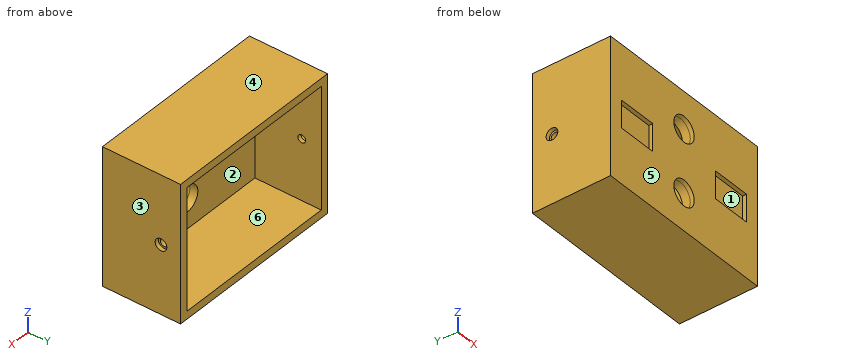
```python
from build123d import *

# Parameters (mm, degrees)
F0_W      = 47
F0_H      = 35
F1_DEPTH  = 19
F2_T      = -2
F3_R      = 3.25
F4_DEPTH  = 19.001
F1_FACE_W = 47
F1_FACE_H = 35
F1_FACE_R = 3.25
F5_DEPTH  = 1
F7_R      = 1
F8_DEPTH  = 47.001
F9_R      = 1.5
F10_DEPTH = 1
F11_R     = 1.5
F12_DEPTH = 1
F13_W     = 10
F13_H     = 7
F14_DEPTH = 1


with BuildPart() as f1:
    # F0 (on Front) → F1 (new body)
    with BuildSketch(Plane.XZ):
        Rectangle(F0_W, F0_H)
    extrude(amount=F1_DEPTH)

    # F2
    f2_openings = [f1.faces().sort_by_distance(p)[0] for p in [
        (0, 0, 0),
    ]]
    offset(amount=F2_T, openings=f2_openings)

    # F3 (on face) → F4 (cut, through all)
    with BuildSketch(Plane.XZ.offset(19)):
        with Locations((0, 8)):
            Circle(F3_R)
        with Locations((0, -8)):
            Circle(F3_R)
    extrude(amount=-F4_DEPTH, mode=Mode.SUBTRACT)

    # F1_face (on face) → F5 (join)
    with BuildSketch(Plane.XZ.offset(19)):
        Rectangle(F1_FACE_W, F1_FACE_H)
        with Locations((0, -8)):
            Circle(F1_FACE_R, mode=Mode.SUBTRACT)
        with Locations((0, 8)):
            Circle(F1_FACE_R, mode=Mode.SUBTRACT)
    extrude(amount=F5_DEPTH)

    # F7 (on face) → F8 (cut, through all)
    with BuildSketch(Plane(origin=(-23.5, 0, 0), x_dir=(0, -1, 0), z_dir=(-1, 0, 0))):
        with Locations((5, 0)):
            Circle(F7_R)
    extrude(amount=-F8_DEPTH, mode=Mode.SUBTRACT)

    # F9 (on face) → F10 (cut)
    with BuildSketch(Plane(origin=(-23.5, 0, 0), x_dir=(0, -1, 0), z_dir=(-1, 0, 0))):
        with Locations((5, 0)):
            Circle(F9_R)
    extrude(amount=-F10_DEPTH, mode=Mode.SUBTRACT)

    # F11 (on face) → F12 (cut)
    with BuildSketch(Plane.YZ.offset(23.5)):
        with Locations((-5, 0)):
            Circle(F11_R)
    extrude(amount=-F12_DEPTH, mode=Mode.SUBTRACT)

    # F13 (on face) → F14 (cut)
    with BuildSketch(Plane.XZ.offset(20)):
        with Locations((-15, 0)):
            Rectangle(F13_W, F13_H)
        with Locations((15, 0)):
            Rectangle(F13_W, F13_H)
    extrude(amount=-F14_DEPTH, mode=Mode.SUBTRACT)


solid = f1.part
```
Can you work these out from the model? Positions are in its coordinate system, mm. Face numbers are marked on the shaded views. A direction names the side the tool comes from. Coordinates: 2 decimals unless noted, no trailing zeros. Write each loop counter-clockwise with the first axis right and the second up, starting at its lowest first coordinate (ties: lowest second). Pieces come first, ordered by that corner, then holes. Notation, with made-up numbers: (72.25, -1.5) - (93.25, -1.5) arc R18 cw to (93.25, 2.5) - close; hole circle Ø3 at (-7.75, 39). An arc over 180 degrees is marked (long way). Return JSON: item names as keys, results as strings.
Q1. Please list where these lines run through material, in increasing order: L1, parallel to Z at x = -5.5, y = -2.25; L2, parallel to Z at x = 22.15, y = -5; L3, parallel to X at y = -12.75, z = -7. Write a range as from..to.
Computed values:
{"L1": "z = -17.5..-15.5, 15.5..17.5", "L2": "z = -17.5..-1, 1..17.5", "L3": "x = -23.5..-21.5, 21.5..23.5"}
Q2. If we section it at A-A (y = -5): Please give me the cut outline in (x, z), then the cut area to 3 significant figures.
Computed values:
{"outline": "(-23.5, -17.5) - (23.5, -17.5) - (23.5, -1.5) - (22.5, -1.5) - (22.5, -1) - (21.5, -1) - (21.5, -15.5) - (-21.5, -15.5) - (-21.5, -1) - (-22.5, -1) - (-22.5, -1.5) - (-23.5, -1.5) - close; (-23.5, 1.5) - (-22.5, 1.5) - (-22.5, 1) - (-21.5, 1) - (-21.5, 15.5) - (21.5, 15.5) - (21.5, 1) - (22.5, 1) - (22.5, 1.5) - (23.5, 1.5) - (23.5, 17.5) - (-23.5, 17.5) - close", "area": "302 mm2"}
Q3. I'm going to push flat-ended pins straight in: pin 1 Ø2.5 at (y, z) = (-5, 0) entering from -X; pin 2 Ø2.5 at (y, z) = (-5, 0) entering from +X; pin 3 Ø2 at (x, z) = (16.5, -1.5) entering from -Y; pin 4 Ø2 at (x, z) = (-1.5, 6.5) entering from -Y. Where does each tip first touch, or does it pass through?
Computed values:
{"pin 1": "stops at x = -22.5", "pin 2": "stops at x = 22.5", "pin 3": "stops at y = -19", "pin 4": "passes through"}
Q4. If we section it at D-D (z = 8): Please give me the cut outline in (x, y).
Computed values:
{"outline": "(-23.5, -20) - (-3.25, -20) - (-3.25, -17) - (-21.5, -17) - (-21.5, 0) - (-23.5, 0) - close; (3.25, -20) - (23.5, -20) - (23.5, 0) - (21.5, 0) - (21.5, -17) - (3.25, -17) - close"}
Q5. If we section it at C-C (z = 2.5): Please give me the cut outline in (x, y), then the cut area to 3 significant figures.
Computed values:
{"outline": "(-23.5, -20) - (-20, -20) - (-20, -19) - (-10, -19) - (-10, -20) - (10, -20) - (10, -19) - (20, -19) - (20, -20) - (23.5, -20) - (23.5, 0) - (21.5, 0) - (21.5, -17) - (-21.5, -17) - (-21.5, 0) - (-23.5, 0) - close", "area": "189 mm2"}
Q6. Thinking about a two-plate mould opening in Z: for the marked faces 4, 5 and 6, which applies, +Z half, -Z half, draft (parallel to the pull), parting line (faces both ways), or undercut?
Computed values:
{"face 4": "+Z half", "face 5": "draft", "face 6": "undercut"}
Q7. If we section it at B-B (x = 0): Please give me the cut outline in (y, z).
Computed values:
{"outline": "(-20, -17.5) - (0, -17.5) - (0, -15.5) - (-17, -15.5) - (-17, -11.25) - (-20, -11.25) - close; (-20, -4.75) - (-17, -4.75) - (-17, 4.75) - (-20, 4.75) - close; (-20, 11.25) - (-17, 11.25) - (-17, 15.5) - (0, 15.5) - (0, 17.5) - (-20, 17.5) - close"}
Q8. On a 3-axis mill with a long thin cutter (end or side, diameter ignored), from which of +Z, -Z, +X, -X, +Y, -Y can I reach the whole of each face in a straight line? I mean the marked faces 1, 2 and 3. Say none if no direction works.
Computed values:
{"face 1": "-Y", "face 2": "+Y", "face 3": "+Z, -Z, +X, +Y, -Y"}
